Verification items for the finished model (mm, model axes). Face numbers are marked on the shaded views. Coordinates: 2 decimals unless noted, no trailing zeros. Order: outer loops, then holes, each group sorted by start corner. A loop starts at its lowest first (then second) coordinate and runs counter-clockwise, first axis right, second up. Notation, with made-up numbers: M -39,21.5 L -13,21.5 A21 ccw -13,33.5 Z; hole C 71,-18.5 d6. An arc over 180 degrees is marked long. Return JSON: item names as keys, results as strings. Group by question number.
Q1. Section check B-B, the plane x = 43. Enter the section's corners in (y, z), then the cut area to 3 significant figures.
Q2. Mould release check, pull along Y, two halves, no side actions. Record for the marked faces 1, 2, 3 and 4: pulls with the +Y half, pulls with the -Y half, needs draft (parallel to the pull), parting line crosses it, or undercut.
Q3. Section check A-A, the plane z = 31. Enter the section's corners in (x, y).
Q4. Thickness scan on probe 1 along X at (y, z) = (-38.5, 18.5); probe 2 along X at (y, z) = (-34, 39); probe 3 along X at (y, z) = (-20.5, 29.5). Record the ranges inside material, lowest first.
Q5. Section check C-C, the plane y = -64.5. Enter the section's corners in (x, z), then the cut area to 3 significant figures.
Q6. Section check D-D, the plane z = -13.5. Enter the section's corners in (x, y).
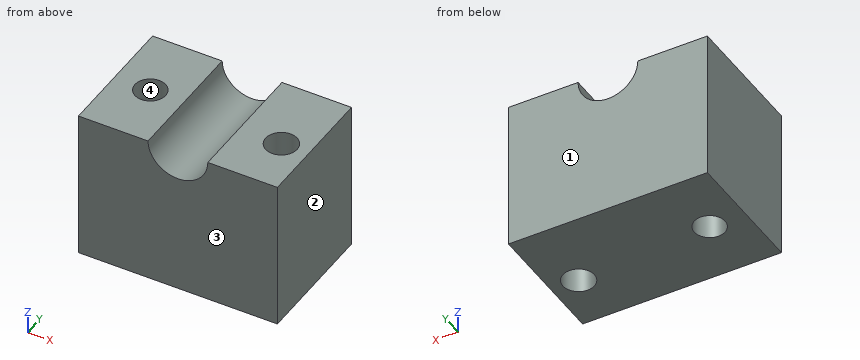
from build123d import *

# Parameters (mm, degrees)
F0_W     = 117.912918
F0_H     = 89.618679
F1_DEPTH = 76.2
F2_R     = 9.121571
F4_DEPTH = 89.619679
F3_R     = 9.352292
F5_DEPTH = 89.619679
F7_DEPTH = 76.201


with BuildPart() as f1:
    # F0 (on Front) → F1 (new body)
    with BuildSketch(Plane.XZ):
        with Locations((0.175312, 0.850113)):
            Rectangle(F0_W, F0_H)
    extrude(amount=F1_DEPTH)

    # F2 (on face) → F4 (cut, through all)
    with BuildSketch(Plane.XY.offset(45.659453)):
        with Locations((-37.546594, -39.185531)):
            Circle(F2_R)
    extrude(amount=-F4_DEPTH, mode=Mode.SUBTRACT)

    # F3 (on face) → F5 (cut, through all)
    with BuildSketch(Plane.XY.offset(45.659453)):
        with Locations((42.910393, -43.953352)):
            Circle(F3_R)
    extrude(amount=-F5_DEPTH, mode=Mode.SUBTRACT)

    # F6 (on face) → F7 (cut, through all)
    with BuildSketch(Plane.XZ.offset(76.2)):
        with BuildLine():
            ThreePointArc((-17.547329, 45.659453), (0.175312, 27.936811), (17.897953, 45.659453))
            Line((17.897953, 45.659453), (-17.547329, 45.659453))
        make_face()
    extrude(amount=-F7_DEPTH, mode=Mode.SUBTRACT)


solid = f1.part
Numbers:
{
 "1": {"outline": "M -76.2,-43.96 L -53.31,-43.96 L -53.31,45.66 L -76.2,45.66 Z; M -34.6,-43.96 L 0,-43.96 L 0,45.66 L -34.6,45.66 Z", "area": "5,150 mm2"},
 "2": {"face 1": "pulls with the +Y half", "face 2": "needs draft", "face 3": "pulls with the -Y half", "face 4": "undercut"},
 "3": {"outline": "M -58.78,-76.2 L -9.78,-76.2 L -9.78,0 L -58.78,0 Z; M 10.13,-76.2 L 59.13,-76.2 L 59.13,0 L 10.13,0 Z; hole C -37.55,-39.19 d18.24; hole C 42.91,-43.95 d18.7"},
 "4": {"probe 1": "x = -58.78 to -46.64, -28.45 to 35.31, 50.51 to 59.13", "probe 2": "x = -58.78 to -45.05, -30.04 to -16.25, 16.6 to 59.13", "probe 3": "x = -58.78 to -7.1, 7.45 to 59.13"},
 "5": {"outline": "M -58.78,-43.96 L 59.13,-43.96 L 59.13,45.66 L 17.9,45.66 A17.72 cw -17.55,45.66 L -58.78,45.66 Z", "area": "10,100 mm2"},
 "6": {"outline": "M -58.78,-76.2 L 59.13,-76.2 L 59.13,0 L -58.78,0 Z; hole C -37.55,-39.19 d18.24; hole C 42.91,-43.95 d18.7"}
}
